The model under review builds one solid part; all positions refer to its coordinate system, in mm. A direction names the side the tool comes from. Coordinates: 2 decimals unless noted, no trailing zeros. Order: outer loops, then holes, each group sorted by start corner. A loop starts at its lowest first (then second) coordinate and runs counter-clockwise, first axis right, second up. Notation, with made-up numbers: (-20.75, 25) -> (38.25, 25) arc R29 ccw to (38.25, 59) -> close; hole circle Ø10 at (59.25, 10.25). An arc over 180 degrees is marked (long way). Use one line per item in the form item = value.
Autodesk Inventor part; units mm, degrees
ref_plane "YZ Plane" through (0, 0, 0) normal (1, 0, 0) x (0, 1, 0)
ref_plane "XZ Plane" through (0, 0, 0) normal (0, 1, 0) x (-1, 0, 0)
ref_plane "XY Plane" through (0, 0, 0) normal (0, 0, 1) x (1, 0, 0)
sketch "Sketch1" plane through (0, 0, 0) normal (0, 1, 0) x (-1, 0, 0)
  circle A0 centre (0, 0) radius 31.75
  line L0 (0, 0) -> (23.8252, 0)
  circle A1 centre (23.8252, 0) radius 2.6162
  circle A2 centre (11.9126, 20.6332) radius 2.6162
  circle A3 centre (-11.9126, 20.6332) radius 2.6162
  circle A4 centre (-23.8252, 0) radius 2.6162
  circle A5 centre (-11.9126, -20.6332) radius 2.6162
  circle A6 centre (11.9126, -20.6332) radius 2.6162
  dimension "d0" = 63.5
  dimension "d1" = 23.8252
  dimension "d2" = 5.2324
  dimension "d5" = 360
extrude "Plate1" add sketch "Sketch1" along normal blind 3.175
sketch "Sketch2" plane through (0, 3.175, 0) normal (0, 1, 0) x (1, 0, 0)
  circle A0 centre (0, 0) radius 31.75
  circle A1 centre (0, 0) radius 4.7625
  line L0 (0, 4.7625) -> (0, 4.2799)
  line L1 (1.1906, 4.2799) -> (1.1906, 4.6113)
  line L2 (-1.1906, 4.2799) -> (-1.1906, 4.6113)
  line L3 (0, 4.7625) -> (0, 5.9531)
  line L4 (0, 5.9531) -> (1.1906, 5.9531)
  line L5 (1.1906, 5.9531) -> (1.1906, 4.6113)
  line L6 (0, 5.9531) -> (-1.1906, 5.9531)
  line L7 (-1.1906, 5.9531) -> (-1.1906, 4.6113)
  dimension "d8" = 9.525
  dimension "d9" = 0.4826
  dimension "d10" = 1.1906
  dimension "d11" = 2.3813
  dimension "d12" = 1.1906
extrude "Cut1" cut sketch "Sketch2" against normal blind 3.175 contours A1 | A1 L3 L4 L5 | L7 L6 L3 A1
equation "\"d13\" = Thickness"
equation "\"BendRadius\" = Thickness"
equation "\"BendReliefWidth\" = Thickness"
equation "\"BendReliefDepth\" = 0.5 * Thickness"
equation "\"CornerReliefSize\" = 4 * Thickness"
equation "\"MinimumRemnant\" = 2 * Thickness"
equation "\"TransitionRadius\" = BendRadius"
equation "\"JacobiRadiusSize\" = BendRadius"
equation "\"GapSize\" = Thickness"
equation "\"d7\" = BendRadius"
properties part number "Fitting piece for Sprocket"
Item 1: We need section A-A (z = 0). State how many separate pieces and enclosed holes the cut face has, plus the area to 3 significant figures.
Results found:
separate_pieces = 4
enclosed_holes = 0
area = 138 mm²
Item 2: To check wall thickness, follow L1, parallel to X at y = 2.2, z = 19; L2, parallel to X at y = 2.5, z = -19.5; L3, parallel to Z at x = -11, y = 1.1. State the ranges of each line that lie inside material, in increasing order. Write a range as from..to.
Results found:
L1 = -25.44..-13.96, -9.87..9.87, 13.96..25.44
L2 = -25.06..-14.27, -9.55..9.55, 14.27..25.06
L3 = -29.78..-23.09, -18.18..18.18, 23.09..29.78
Item 3: Tool access review of faces 1 (the face through (0, 2, -5.953)), 2 (the face through (0, 0, -7)): name each direction out of +Z, -Z, +X, -X, +Y, -Y from which nothing blocks a thin tool from reaching the whole face with its end or side.
Results found:
face_1 = +Y, -Y
face_2 = +Z, -Z, +X, -X, -Y
Item 4: Draft analysis for pull direction X (two halves, no side actions). For faces 3 (the face through (9.496, 1.565, -19.631)), 4 (the face through (6.883, 1.565, 30.995)), 5 (the face through (0, 3.175, -7)), state which applies: released by +X, released by -X, zero draft, split by the parting line, or undercut.
Results found:
face_3 = undercut
face_4 = split by the parting line
face_5 = zero draft
Item 5: We need section D-D (x = 24). Write out the cut boundary in (y, z) (3 decimals).
Results found:
outline = (0, -20.786) -> (3.175, -20.786) -> (3.175, -2.61) -> (0, -2.61) -> close; (0, 2.61) -> (3.175, 2.61) -> (3.175, 20.786) -> (0, 20.786) -> close
Item 6: Clearance check with flat-ended pins moving along their axes: pin 1 (4 mm diameter, centred on x = 18, z = -6.5, fed in from -Y); pin 2 (0.7 mm diameter, centred on y = 1.5, z = -5.5, fed in from -X); pin 3 (3 mm diameter, centred on x = -11.91, z = 20.63, fed in from -Y); pin 4 (1.9 mm diameter, centred on x = -0.5, y = 1.5, fed in from +Z). State where each tip first meets the part, or that it passes through.
Results found:
pin_1 = 0
pin_2 = -31.33
pin_3 = through
pin_4 = 31.75
